from build123d import *

# Parameters (mm, degrees)
SKETCH1_W           = 25.4
SKETCH1_H           = 25.4
SKETCH1_W_2         = 23.4696
SKETCH1_H_2         = 23.4696
BOSS_EXTRUDE1_DEPTH = 327.152
SKETCH3_R           = 3.175
CUT_EXTRUDE1_DEPTH  = 292.1


with BuildPart() as part:
    # Sketch1 → Boss-Extrude1 (new body)
    with BuildSketch(Plane(origin=(0, 0, 0), x_dir=(1, 0, 0), z_dir=(0, 1, 0))):
        Rectangle(SKETCH1_W, SKETCH1_H)
        Rectangle(SKETCH1_W_2, SKETCH1_H_2, mode=Mode.SUBTRACT)
    extrude(amount=BOSS_EXTRUDE1_DEPTH)

    # Sketch3 → Cut-Extrude1 (cut)
    with BuildSketch(Plane.XY.offset(12.7)):
        with Locations((0, 12.7)):
            Circle(SKETCH3_R)
    extrude(amount=-CUT_EXTRUDE1_DEPTH, mode=Mode.SUBTRACT)


solid = part.part
Design review of the part built by this model. Coordinates are the model's own, in mm. A direction names the side the tool comes from. Coordinates: 2 decimals unless noted, no trailing zeros. Order: outer loops, then holes, each group sorted by start corner. A loop starts at its lowest first (then second) coordinate and runs counter-clockwise, first axis right, second up. Notation, with made-up numbers: M -37.75,0.25 L -11.75,0.25 A18 ccw -11.75,6.25 Z; hole C 27,-4 d3. An arc over 180 degrees is marked long. Use a Markdown table: item, result.
(1) Add section D-D (y = 12.7). Give the boundary of the cut face in (x, z) (3 decimals), then the cut area to 3 significant figures.
Worked answers:
| item | result |
|---|---|
| outline | M -12.7,-12.7 L -3.175,-12.7 L -3.175,-11.735 L -11.735,-11.735 L -11.735,11.735 L -3.175,11.735 L -3.175,12.7 L -12.7,12.7 Z; M 3.175,-12.7 L 12.7,-12.7 L 12.7,12.7 L 3.175,12.7 L 3.175,11.735 L 11.735,11.735 L 11.735,-11.735 L 3.175,-11.735 Z |
| area | 82.1 mm2 |
(2) For faces 1 (the flat face through (-11.735, 161, 0)), 2 (the cylindrical face through (1.5, 9.9, 12.2)), list the 3-axis set-ups (+Z, -Z, +X, -X, +Y, -Y) from which the entire face can be reached by the end or side of a thin tool; tool diameter is ignored.
Worked answers:
| item | result |
|---|---|
| face 1 | +Y, -Y |
| face 2 | +Z, -Z |
(3) Add section C-C (y = 104). Give the boundary of the cut face in (x, z).
Worked answers:
| item | result |
|---|---|
| outline | M -12.7,-12.7 L 12.7,-12.7 L 12.7,12.7 L -12.7,12.7 Z; hole M -11.73,-11.73 L 11.73,-11.73 L 11.73,11.73 L -11.73,11.73 Z |
(4) Add section A-A (x = 0). Give the boundary of the cut face in (y, z) (3 decimals).
Worked answers:
| item | result |
|---|---|
| outline | M 0,-12.7 L 9.525,-12.7 L 9.525,-11.735 L 0,-11.735 Z; M 0,11.735 L 9.525,11.735 L 9.525,12.7 L 0,12.7 Z; M 15.875,-12.7 L 327.152,-12.7 L 327.152,-11.735 L 15.875,-11.735 Z; M 15.875,11.735 L 327.152,11.735 L 327.152,12.7 L 15.875,12.7 Z |
(5) Draft analysis for pull direction X (two halves, no side actions). For faces 3 (the flat face through (-12.7, 161, 0)), 4 (the flat face through (-1, 327.152, 12)), 5 (the flat face through (0, 161, 11.735)), state which applies: released by +X, released by -X, zero draft, split by the parting line, or undercut.
Worked answers:
| item | result |
|---|---|
| face 3 | released by -X |
| face 4 | zero draft |
| face 5 | undercut |
(6) Wall thickness on probe 1 along Y at (x, z) = (0, -12) (3 decimals); probe 2 along X at (y, z) = (173, -1.25): over which ranges is each line inside the solid? List them lowest first.
Worked answers:
| item | result |
|---|---|
| probe 1 | y = 0 to 9.525, 15.875 to 327.152 |
| probe 2 | x = -12.7 to -11.73, 11.73 to 12.7 |
(7) Add section B-B (z = 8.5). Give the boundary of the cut face in (x, y).
Worked answers:
| item | result |
|---|---|
| outline | M -12.7,0 L -11.73,0 L -11.73,327.15 L -12.7,327.15 Z; M 11.73,0 L 12.7,0 L 12.7,327.15 L 11.73,327.15 Z |
